from build123d import *

# Parameters (mm, degrees)
SKETCH1_W           = 36.83
SKETCH1_H           = 34.29
BOSS_EXTRUDE1_DEPTH = 3.81
SKETCH2_W           = 1.016
SKETCH2_H           = 34.29
BOSS_EXTRUDE2_DEPTH = 1.27
FILLET1_R           = 0.254
SKETCH3_R           = 3.81
SKETCH3_R_2         = 1.27
CUT_EXTRUDE1_DEPTH  = 3.81
CHAMFER1_SIZE       = 2.54


with BuildPart() as part:
    # Sketch1 → Boss-Extrude1 (new body)
    with BuildSketch(Plane.XY):
        Rectangle(SKETCH1_W, SKETCH1_H)
    extrude(amount=BOSS_EXTRUDE1_DEPTH)

    # Sketch2 → Boss-Extrude2 (add)
    with BuildSketch(Plane(origin=(18.415, 0, 0), x_dir=(0, 0, -1), z_dir=(1, 0, 0))):
        with Locations((-1.778, 0)):
            Rectangle(SKETCH2_W, SKETCH2_H)
    boss_extrude2 = extrude(amount=BOSS_EXTRUDE2_DEPTH)

    # Mirror1: Boss-Extrude2 across plane
    add(boss_extrude2.mirror(Plane(origin=(0, 0, 0), x_dir=(0, 0, 1), z_dir=(1, 0, 0))))

    # Fillet1
    fillet1_edges = [part.edges().sort_by_distance(p)[0] for p in [
        (19.685, 0, 2.286),
        (19.685, 0, 1.27),
        (-19.685, 0, 2.286),
        (-19.685, 0, 1.27),
    ]]
    fillet(fillet1_edges, radius=FILLET1_R)

    # Sketch3 → Cut-Extrude1 (cut)
    with BuildSketch(Plane.XY.offset(3.81)):
        with Locations((0, -1.905)):
            Circle(SKETCH3_R)
        with Locations((-11.176, 9.271)):
            Circle(SKETCH3_R_2)
        with Locations((11.176, 9.271)):
            Circle(SKETCH3_R_2)
        with Locations((11.176, -13.081)):
            Circle(SKETCH3_R_2)
        with Locations((-11.176, -13.081)):
            Circle(SKETCH3_R_2)
    extrude(amount=-CUT_EXTRUDE1_DEPTH, mode=Mode.SUBTRACT)

    # Chamfer1
    chamfer1_edges = [part.edges().sort_by_distance(p)[0] for p in [
        (0, 17.145, 0),
    ]]
    chamfer(chamfer1_edges, length=CHAMFER1_SIZE)


solid = part.part
Geometry check sheet. Reference: the model listing, model coordinates, mm. A direction names the side the tool comes from. Round coordinates to 2 decimals unless told otherwise and drop trailing zeros. Order: outer loops, then holes, each group sorted by start corner. A loop starts at its lowest first (then second) coordinate and runs counter-clockwise, first axis right, second up. Notation, with made-up numbers: M -37.75,17 L 10.25,17 A9 ccw 10.25,30 Z; hole C 43.5,-25.5 d1. An arc over 180 degrees is marked long. Answer in a Markdown table with one row per item. Add a question column.
Item 1: Set-up check for faces 5 (the face through (18.415, 0, 3)), 6 (the face through (-19, 0, 2.286)), 7 (the face through (19, -1, 1.27)), 8 (the face through (-19, -1, 1.27)): record each of +Z, -Z, +X, -X, +Y, -Y from which the full face is reachable in a straight line by a thin tool's end or side.
Item 2: Sectioned sample at B-B, the plane y = -8.5. Enter the section's corners in (x, z) (3 decimals), plus the area to 3 significant figures.
Item 3: Sectioned sample at A-A, the plane x = 0. Enter the section's corners in (y, z) (3 decimals).
Item 4: Sectioned sample at D-D, the plane z = 0.85. Enter the section's corners in (x, y) (3 decimals).
Item 5: Draft check along Y on faces 1 (the face through (12.35, -13.57, 1.93)), 2 (the face through (-18.415, -1, 1)), 3 (the face through (0, -17.145, 2)), 4 (the face through (0, 17.145, 3)). Enter one of: released by +Y, released by -Y, zero draft, split by the parting line, or undercut.
Item 6: Depth check by flat-ended pin: pin 1 Ø1.7 at (y, z) = (-3.5, 3) entering from +X; pin 2 Ø0.8 at (x, y) = (-19, 6) entering from -Z; pin 3 Ø0.5 at (x, y) = (19, 0.5) entering from +Z. Enter the tip coordinate at first touch or a pass-through.
Item 7: Sectioned sample at C-C, the plane y = -2.5. Enter the section's corners in (x, z) (3 decimals), plus the area to 3 significant figures.
Item 8: Material ranges on L1, parallel to X at y = -12, z = 0.6 (3 decimals); L2, parallel to Y at x = -11.5, z = 3.25 (3 decimals); L3, parallel to X at y = -12.5, z = 1.65 (3 decimals), recorded low to high. Write a range as [from, to].
Filled in:
| question | item | result |
|---|---|---|
| 1 | face 5 | +Z, +X, +Y, -Y |
| 1 | face 6 | +Z, -X, +Y, -Y |
| 1 | face 7 | -Z, +X, +Y, -Y |
| 1 | face 8 | -Z, -X, +Y, -Y |
| 2 | outline | M -19.685,1.524 A0.254 ccw -19.431,1.27 L -18.415,1.27 L -18.415,0 L 18.415,0 L 18.415,1.27 L 19.431,1.27 A0.254 ccw 19.685,1.524 L 19.685,2.032 A0.254 ccw 19.431,2.286 L 18.415,2.286 L 18.415,3.81 L -18.415,3.81 L -18.415,2.286 L -19.431,2.286 A0.254 ccw -19.685,2.032 Z |
| 2 | area | 143 mm² |
| 3 | outline | M -17.145,0 L -5.715,0 L -5.715,3.81 L -17.145,3.81 Z; M 1.905,0 L 14.605,0 L 17.145,2.54 L 17.145,3.81 L 1.905,3.81 Z |
| 4 | outline | M -18.415,-17.145 L 18.415,-17.145 L 18.415,15.455 L -18.415,15.455 Z; hole C -11.176,-13.081 d2.54; hole C -11.176,9.271 d2.54; hole C 0,-1.905 d7.62; hole C 11.176,-13.081 d2.54; hole C 11.176,9.271 d2.54 |
| 5 | face 1 | undercut |
| 5 | face 2 | zero draft |
| 5 | face 3 | released by -Y |
| 5 | face 4 | released by +Y |
| 6 | pin 1 | stops at x = 19.66 |
| 6 | pin 2 | stops at z = 1.27 |
| 6 | pin 3 | stops at z = 2.29 |
| 7 | outline | M -19.685,1.524 A0.254 ccw -19.431,1.27 L -18.415,1.27 L -18.415,0 L -3.763,0 L -3.763,3.81 L -18.415,3.81 L -18.415,2.286 L -19.431,2.286 A0.254 ccw -19.685,2.032 Z; M 3.763,0 L 18.415,0 L 18.415,1.27 L 19.431,1.27 A0.254 ccw 19.685,1.524 L 19.685,2.032 A0.254 ccw 19.431,2.286 L 18.415,2.286 L 18.415,3.81 L 3.763,3.81 Z |
| 7 | area | 114 mm² |
| 8 | L1 | x = [-18.415, -11.843], [-10.509, 10.509], [11.843, 18.415] |
| 8 | L2 | y = [-17.145, -14.309], [-11.853, 8.043], [10.499, 17.145] |
| 8 | L3 | x = [-19.685, -12.305], [-10.047, 10.047], [12.305, 19.685] |
